Read the model definition and answer for the solid it produces. Units are mm, in the model's axes. A direction names the side the tool comes from. Round coordinates to 2 decimals unless told otherwise and drop trailing zeros. Return JSON: item names as keys, results as strings. Group by question number.
(1) Straight lines are drawn through the part: line 1 (X direction, y = 2.75, z = -4.25); line 2 (Z direction, x = -4.75, y = 2.5); line 3 (X direction, y = 7, z = -2). For each, find the intervals that lie inside material, in ascending order.
(2) For faces 1 (the flat face through (1.71, 4.44, 4.71)), 2 (the flat face through (4.901, 4.437, -1.022)), 3 (the flat face through (1.714, 4.437, -4.688)), 4 (the flat face through (-4.98, 4.44, 0.39)), determine the directions among +Z, -Z, +X, -X, +Y, -Y from which every point of the face is accessible in a straight line to the end or side of a thin tool.
(3) Given pin 1 (1 mm diameter, centred on x = 1.5, z = 4, fed in from -Y); pin 2 (5 mm diameter, centred on x = -4, y = 7.5, fed in from +Z); pin 3 (2 mm diameter, centred on y = 1, z = -2.5, fed in from +X); pin 4 (1.5 mm diameter, centred on x = 0.5, z = -1.5, fed in from -Y), each flat-ended and moving along its own axis, determine where each tip first touches the part or whether it passes through.
(4) The mould has two halves that part along X. Classify faces 5 (the flat face through (-4.99, 4.44, -0.4)), 6 (the flat face through (1.106, 4.437, -4.883)), 7 (the flat face through (3.976, 4.437, -3.018)): released by +X, released by -X, zero draft, split by the parting line, or undercut.
```python
from build123d import *

# Parameters (mm, degrees)
SKETCH1_R           = 2.5
BOSS_EXTRUDE1_DEPTH = 9


with BuildPart() as part:
    # Sketch1 → Boss-Extrude1 (new body)
    with BuildSketch(Plane(origin=(0, 0, 0), x_dir=(1, 0, 0), z_dir=(0, 1, 0))):
        Polygon((1.561153305, 5.316799887), (0.637864624, 4.436445909), (0, 5.541259846), (-0.637864624, 4.436445909), (-1.561153305, 5.316799887), (-1.861917874, 4.077031446), (-2.995831253, 4.661604422), (-2.935129611, 3.387320142), (-4.18780477, 3.62875349), (-3.770554603, 2.423188306), (-5.040507251, 2.301922531), (-4.300511685, 1.262744164), (-5.484857811, 0.788603499), (-4.482066887, 0), (-5.484857811, -0.788603499), (-4.300511685, -1.262744164), (-5.040507251, -2.301922531), (-3.770554603, -2.423188306), (-4.18780477, -3.62875349), (-2.935129611, -3.387320142), (-2.941213111, -3.515028519), (-2.995831253, -4.661604422), (-1.861917874, -4.077031446), (-1.561153305, -5.316799887), (-0.637864624, -4.436445909), (0, -5.541259846), (0.637864624, -4.436445909), (1.561153305, -5.316799887), (1.861917874, -4.077031446), (2.995831253, -4.661604422), (2.935129611, -3.387320142), (4.18780477, -3.62875349), (3.770554603, -2.423188306), (5.040507251, -2.301922531), (4.300511685, -1.262744164), (5.484857811, -0.788603499), (4.482066887, 0), (5.484857811, 0.788603499), (4.300511685, 1.262744164), (5.040507251, 2.301922531), (3.770554603, 2.423188306), (4.18780477, 3.62875349), (3.001290377, 3.400071585), (2.935129611, 3.387320142), (2.941213111, 3.515028519), (2.995831253, 4.661604422), (1.861917874, 4.077031446), align=None)
        Circle(SKETCH1_R, mode=Mode.SUBTRACT)
    extrude(amount=BOSS_EXTRUDE1_DEPTH)


solid = part.part
```
Checks:
{
 "1": {"line 1": "x = -2.98 to -2.2, -1.82 to 1.82, 2.2 to 2.98", "line 2": "z = -2.33 to -1.89, -1.08 to -0.21, 0.21 to 1.08, 1.89 to 2.33", "line 3": "x = -4.83 to -1.5, 1.5 to 4.83"},
 "2": {"face 1": "+Z, +Y, -Y", "face 2": "+X, +Y, -Y", "face 3": "-Z, +Y, -Y", "face 4": "-X, +Y, -Y"},
 "3": {"pin 1": "stops at y = 0", "pin 2": "stops at z = 5.32", "pin 3": "stops at x = 5.04", "pin 4": "passes through"},
 "4": {"face 5": "released by -X", "face 6": "undercut", "face 7": "released by +X"}
}
